from build123d import *

# Parameters (mm, degrees)
EXTRUDE_1_DEPTH = 5


with BuildPart() as part:
    # 草图2 → 凸台-拉伸1 (new body)
    # profile 1 of 2: a face of its own
    with BuildSketch(Plane(origin=(0, 0, 0), x_dir=(0, 0, -1), z_dir=(1, 0, 0))):
        with BuildLine():
            ThreePointArc((-52, -6.305745823), (-50, -4.305745823), (-48, -6.305745823))
            Line((-48, -6.305745823), (-27, -6.305745823))
            ThreePointArc((-27, -6.305745823), (-25, -4.305745823), (-23, -6.305745823))
            Line((-23, -6.305745823), (-2, -6.305745823))
            ThreePointArc((-2, -6.305745823), (0, -4.305745823), (2, -6.305745823))
            Line((2, -6.305745823), (23, -6.305745823))
            ThreePointArc((23, -6.305745823), (25, -4.305745823), (27, -6.305745823))
            Line((27, -6.305745823), (48, -6.305745823))
            ThreePointArc((48, -6.305745823), (50, -4.305745823), (52, -6.305745823))
            Line((52, -6.305745823), (60, -6.305745823))
            Line((60, -6.305745823), (60, 10))
            Line((60, 10), (-60, 10))
            Line((-60, 10), (-60, -6.305745823))
            Line((-60, -6.305745823), (-52, -6.305745823))
        make_face()
        with BuildLine():
            Line((55, -1.09255297), (-55, -1.09255297))
            ThreePointArc((-55, -1.09255297), (-57, 0.90744703), (-55, 2.90744703))
            Line((-55, 2.90744703), (55, 2.90744703))
            ThreePointArc((55, 2.90744703), (57, 0.90744703), (55, -1.09255297))
        make_face(mode=Mode.SUBTRACT)
    # profile 2 of 2: a face of its own
    with BuildSketch(Plane(origin=(0, 0, 0), x_dir=(0, 0, -1), z_dir=(1, 0, 0))):
        with BuildLine():
            Line((-27, -6.305745823), (-48, -6.305745823))
            ThreePointArc((-48, -6.305745823), (-50, -8.305745823), (-52, -6.305745823))
            Line((-52, -6.305745823), (-60, -6.305745823))
            Line((-60, -6.305745823), (-60, -10))
            Line((-60, -10), (60, -10))
            Line((60, -10), (60, -6.305745823))
            Line((60, -6.305745823), (52, -6.305745823))
            ThreePointArc((52, -6.305745823), (50, -8.305745823), (48, -6.305745823))
            Line((48, -6.305745823), (27, -6.305745823))
            ThreePointArc((27, -6.305745823), (25, -8.305745823), (23, -6.305745823))
            Line((23, -6.305745823), (2, -6.305745823))
            ThreePointArc((2, -6.305745823), (0, -8.305745823), (-2, -6.305745823))
            Line((-2, -6.305745823), (-23, -6.305745823))
            ThreePointArc((-23, -6.305745823), (-25, -8.305745823), (-27, -6.305745823))
        make_face()
    extrude(amount=EXTRUDE_1_DEPTH)


solid = part.part
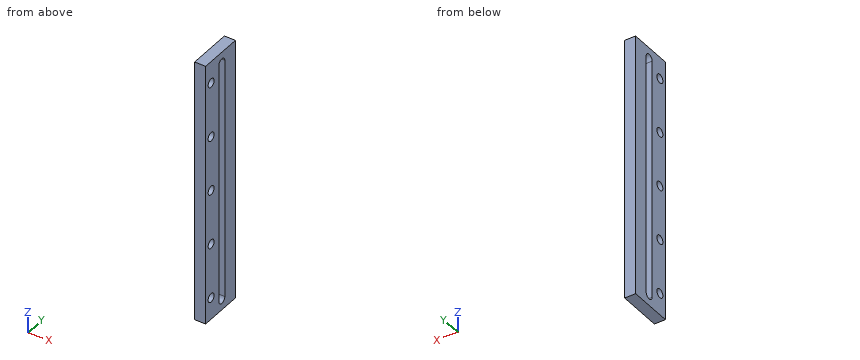
Read the model definition and answer for the solid it produces. Units are mm, in the model's axes. Round coordinates to 2 decimals unless told otherwise and drop trailing zeros. Order: outer loops, then holes, each group sorted by start corner. A loop starts at its lowest first (then second) coordinate and runs counter-clockwise, first axis right, second up.
1) A flat-ended cylindrical pin translates along its axis: pin 1 (4.5 mm diameter, centred on y = -6.31, z = 50, fed in from -X). Find the tip coordinate at first contact, or state that the pin passes through.
2) The part is cut by section C-C on x = 2.5. Write down the section's boundary in (y, z), plus the area to 3 significant figures.
3) Straight lines are drawn through the part: L1, parallel to Z at x = 3.1, y = -6.5; L2, parallel to Y at x = 3.2, z = 50; L3, parallel to Y at x = 2.75, z = 10. For each, find the intervals that lie inside material, in ascending order.
4) The part is cut by section B-B on z = -25. Write down the section's boundary in (x, y), plus the area to 3 significant figures.
5) The part is cut by section A-A on z = -5. Write down the section's boundary in (x, y), plus the area to 3 significant figures.
Resolved:
1. pin 1: stops at x = 0
2. outline: (-10, -60) - (10, -60) - (10, 60) - (-10, 60) - close; hole circle Ø4 at (-6.31, -50); hole circle Ø4 at (-6.31, -25); hole circle Ø4 at (-6.31, 0); hole circle Ø4 at (-6.31, 25); hole circle Ø4 at (-6.31, 50); hole (-1.09, -55) arc R2 ccw to (2.91, -55) - (2.91, 55) arc R2 ccw to (-1.09, 55) - close
2. area: 1,880 mm2
3. L1: z = -60 to -51.99, -48.01 to -26.99, -23.01 to -1.99, 1.99 to 23.01, 26.99 to 48.01, 51.99 to 60
3. L2: y = -10 to -8.31, -4.31 to -1.09, 2.91 to 10
3. L3: y = -10 to -1.09, 2.91 to 10
4. outline: (0, -10) - (5, -10) - (5, -8.31) - (0, -8.31) - close; (0, -4.31) - (5, -4.31) - (5, -1.09) - (0, -1.09) - close; (0, 2.91) - (5, 2.91) - (5, 10) - (0, 10) - close
4. area: 60.0 mm2
5. outline: (0, -10) - (5, -10) - (5, -1.09) - (0, -1.09) - close; (0, 2.91) - (5, 2.91) - (5, 10) - (0, 10) - close
5. area: 80.0 mm2
